Verification items for the finished model (mm, model axes). A direction names the side the tool comes from. Give positions to 0.01 mm unless a question says otherwise; leave off trailing zeros. Loops run counter-clockwise (first coordinate to the right, second up) from the corner with the lowest first, then second, coordinate; pieces in that order, holes last. Notation, with made-up numbers: (-38.5, 22.5) - (-0.5, 22.5) arc R6 cw to (-0.5, 29.5) - close; hole circle Ø3 at (-11.5, 32.5). An arc over 180 degrees is marked (long way). Answer in a Markdown table with one row per item.
```python
from build123d import *

# Parameters (mm, degrees)
SKETCH2_R           = 5
BOSS_EXTRUDE1_DEPTH = 15
BOSS_EXTRUDE2_START = 2
SKETCH3_R           = 5
SKETCH3_R_2         = 0.75
BOSS_EXTRUDE2_DEPTH = 2
SKETCH4_R           = 5
BOSS_EXTRUDE3_DEPTH = 3


with BuildPart() as part:
    # Sketch2 → Boss-Extrude1 (new body)
    with BuildSketch(Plane(origin=(0, 0, 0), x_dir=(1, 0, 0), z_dir=(0, 1, 0))):
        with Locations(Location((0, 0, 0), (0, 0, 270))):
            Circle(SKETCH2_R)
        with BuildLine():
            Line((1.299038106, 0.75), (3.464101615, -0.5))
            ThreePointArc((3.464101615, -0.5), (3.031088913, 1.75), (1.299038106, 3.25))
            Line((1.299038106, 3.25), (1.299038106, 0.75))
        make_face(mode=Mode.SUBTRACT)
        with BuildLine():
            Line((-1.299038106, 0.75), (-1.299038106, 3.25))
            ThreePointArc((-1.299038106, 3.25), (-3.031088913, 1.75), (-3.464101615, -0.5))
            Line((-3.464101615, -0.5), (-1.299038106, 0.75))
        make_face(mode=Mode.SUBTRACT)
        with BuildLine():
            Line((0, -1.5), (-2.165063509, -2.75))
            ThreePointArc((-2.165063509, -2.75), (0, -3.5), (2.165063509, -2.75))
            Line((2.165063509, -2.75), (0, -1.5))
        make_face(mode=Mode.SUBTRACT)
    extrude(amount=BOSS_EXTRUDE1_DEPTH)

    # Sketch3 → Boss-Extrude2 (add)
    with BuildSketch(Plane.XZ.offset(BOSS_EXTRUDE2_START)):
        with Locations(Location((0, 0, 0), (0, 0, 270))):
            Circle(SKETCH3_R)
        with Locations(Location((0, 2.5, 0), (0, 0, 270))):
            Circle(SKETCH3_R_2, mode=Mode.SUBTRACT)
        with Locations(Location((2.165063509, -1.25, 0), (0, 0, 270))):
            Circle(SKETCH3_R_2, mode=Mode.SUBTRACT)
        with Locations(Location((-2.165063509, -1.25, 0), (0, 0, 270))):
            Circle(SKETCH3_R_2, mode=Mode.SUBTRACT)
    extrude(amount=-BOSS_EXTRUDE2_DEPTH)

    # Sketch4 → Boss-Extrude3 (add)
    with BuildSketch(Plane(origin=(0, 15, 0), x_dir=(1, 0, 0), z_dir=(0, 1, 0))):
        with Locations(Location((0, 0, 0), (0, 0, 90))):
            Circle(SKETCH4_R)
    extrude(amount=BOSS_EXTRUDE3_DEPTH)


solid = part.part
```
Q1. Sectioned sample at B-B (z = 0). Record the cut outline in (x, y).
Completed:
| item | result |
|---|---|
| outline | (-5, -2) - (5, -2) - (5, 18) - (-5, 18) - close; hole (-3.5, 0) - (-2.6, 0) - (-2.6, 15) - (-3.5, 15) - close; hole (2.6, 0) - (3.5, 0) - (3.5, 15) - (2.6, 15) - close |
Q2. Tool access check on faces 3 (the face through (0, -2, 0)), 4 (the face through (1.299, 7, -2)), 5 (the face through (1.433, -1.014, -1.087)). Record the directions out of +Z, -Z, +X, -X, +Y, -Y that give a thin tool (end or side, any length) a straight path to the whole face; none if there is none.
Completed:
| item | result |
|---|---|
| face 3 | +Z, -Z, +X, -X, -Y |
| face 4 | none |
| face 5 | -Y |
Q3. Sectioned sample at D-D (y = 16.75). Record the cut outline in (x, z), and give its area (3 significant figures).
Completed:
| item | result |
|---|---|
| outline | circle Ø10 at (0, 0) |
| area | 78.5 mm^2 |
Q4. Sectioned sample at A-A (y = 11). Record the cut outline in (x, z).
Completed:
| item | result |
|---|---|
| outline | circle Ø10 at (0, 0); hole (-3.46, 0.5) arc R3.5 ccw to (-1.3, -3.25) - (-1.3, -0.75) - close; hole (-2.17, 2.75) - (0, 1.5) - (2.17, 2.75) arc R3.5 ccw to start; hole (1.3, -3.25) arc R3.5 ccw to (3.46, 0.5) - (1.3, -0.75) - close |
Q5. Draft check along X on faces 1 (the face through (-2.4, 0, -2.2)), 2 (the face through (0, 18, 0)). Enter one of: +X half, -X half, draft (parallel to the pull), parting line (faces both ways), or undercut.
Completed:
| item | result |
|---|---|
| face 1 | undercut |
| face 2 | draft |
Q6. Sectioned sample at C-C (x = 0.5). Record the cut outline in (y, z).
Completed:
| item | result |
|---|---|
| outline | (-2, -4.97) - (18, -4.97) - (18, 4.97) - (-2, 4.97) - (-2, 3.06) - (0, 3.06) - (0, 3.46) - (15, 3.46) - (15, 1.79) - (0, 1.79) - (0, 1.94) - (-2, 1.94) - close |
Q7. Go/stop test with flat-tipped pins: P1, Ø1.5, axis at y = 15.5, z = -3, coming from the +X side; P2, Ø0.8, axis at y = 4.5, z = -1.5, coming from the -X side; P3, Ø1.2, axis at y = 9.5, z = -2, coming from the +X side. Record where each tip stops, or that it passes through.
Completed:
| item | result |
|---|---|
| P1 | x = 4.47 |
| P2 | x = -4.88 |
| P3 | x = 4.8 |
Q8. Thickness scan on line 1 (X direction, y = -0.65, z = -1.25); line 2 (X direction, y = 8.75, z = -1.75); line 3 (Z direction, x = -1.5, y = 6.5). Record the ranges inside material, lowest first.
Completed:
| item | result |
|---|---|
| line 1 | -4.84 to -2.92, -1.42 to 1.42, 2.92 to 4.84 |
| line 2 | -4.68 to -3.03, -1.3 to 1.3, 3.03 to 4.68 |
| line 3 | -4.77 to -3.16, -0.63 to 2.37, 3.16 to 4.77 |
